Job drawing, mm, ordinate dimensions from the low corner. One solid piece. Coordinates: 2 decimals unless noted, no trailing zeros. Order: outer loops, then holes, each group sorted by start corner. A loop starts at its lowest first (then second) coordinate and runs counter-clockwise, first axis right, second up. Notation, with made-up numbers: (46, -2) - (84, -2) arc R30 cw to (84, 33) - close; hole circle Ø1 at (80, 3.25). An arc over 180 degrees is marked (long way). Use one line per item in the form item = value.
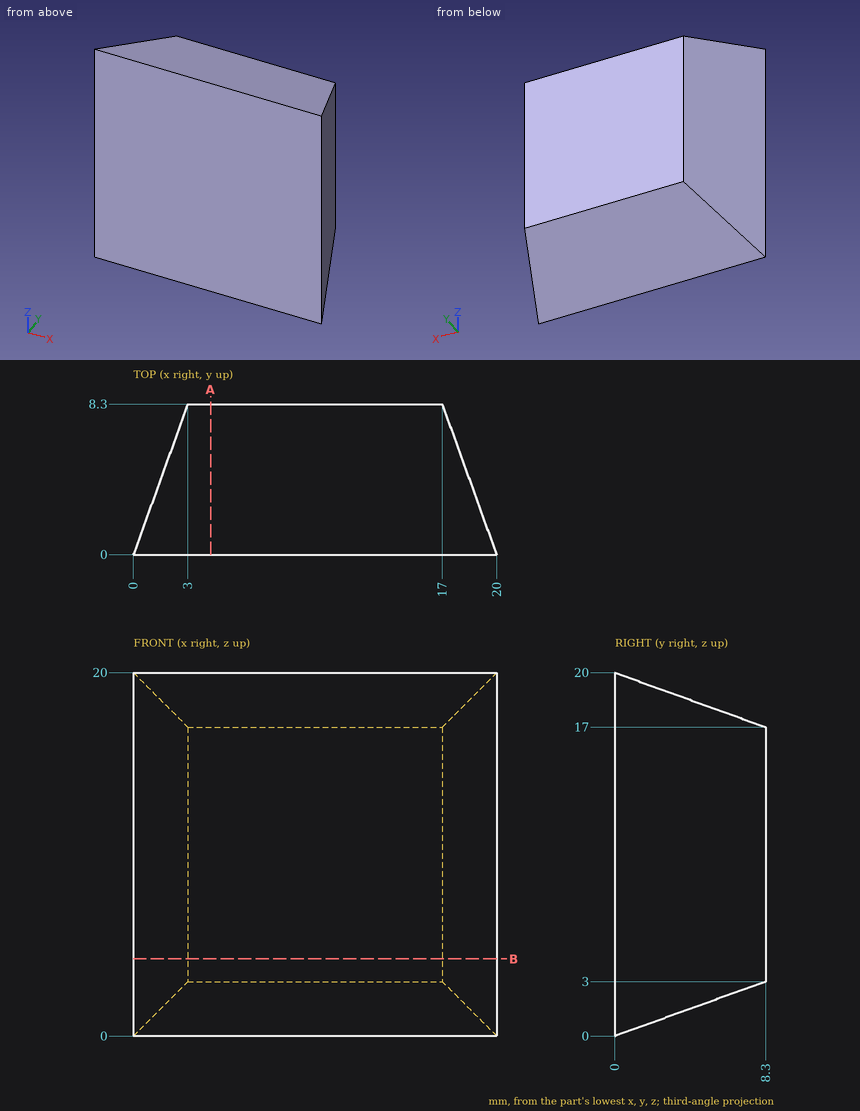
Item 1: Cut at A-A, the plane x = 4.25. Write the cut outline in (y, z).
Derived:
outline = (0, 0) - (8.3, 3) - (8.3, 17) - (0, 20) - close
Item 2: Cut at B-B, the plane z = 4.25. Write the cut outline in (x, y), plus the area to 3 significant figures.
Derived:
outline = (0, 0) - (20, 0) - (17, 8.3) - (3, 8.3) - close
area = 141 mm²
Item 3: Drill centre lines: line 1 (X direction, y = 5.75, z = 4); line 2 (X direction, y = 2.25, z = 17.25); line 3 (Z direction, x = 11, y = 0.5). Where is each one in solid material? Low to high. Write a range as [from, to].
Derived:
line_1 = [2.08, 17.92]
line_2 = [0.81, 19.19]
line_3 = [0.18, 19.82]
Item 4: Drop flat-ended pins along their axis: pin 1 (2 mm diameter, centred on y = 5.5, z = 3, fed in from +X); pin 2 (3 mm diameter, centred on y = 1, z = 18, fed in from +X). Give the stop position or say it passes through.
Derived:
pin_1 = 18.37
pin_2 = 20
